Read the model definition and answer for the solid it produces. Units are mm, in the model's axes. Coordinates: 2 decimals unless noted, no trailing zeros. Write each loop counter-clockwise with the first axis right and the second up, starting at its lowest first coordinate (ties: lowest second). Pieces come first, ordered by that corner, then holes. Notation, with made-up numbers: M 54.25,50 L 78.25,50 A30 ccw 78.25,76 Z; hole C -7,-13 d8. An arc over 180 degrees is marked long. Write item = value, one per line.
Autodesk Inventor part; units mm, degrees
ref_plane "YZ Plane" through (0, 0, 0) normal (1, 0, 0) x (0, 1, 0)
ref_plane "XZ Plane" through (0, 0, 0) normal (0, 1, 0) x (-1, 0, 0)
ref_plane "XY Plane" through (0, 0, 0) normal (0, 0, 1) x (1, 0, 0)
sketch "Sketch1" plane through (0, 0, 0) normal (0, 1, 0) x (-1, 0, 0)
  line L0 (0, 0) -> (245, 0)
  line L1 (245, 0) -> (245, -355.6)
  line L2 (245, -355.6) -> (0, -355.6)
  line L3 (0, -355.6) -> (0, 0)
  line L4 (0, -355.6) -> (67.5, -355.6)
  line L5 (67.5, -355.6) -> (67.5, -280.6)
  line L6 (67.5, -280.6) -> (0, -280.6)
  line L7 (0, -280.6) -> (0, -355.6)
  line L8 (0, 0) -> (67.4878, 0)
  line L9 (67.4878, 0) -> (67.4878, -75.0062)
  line L10 (67.4878, -75.0062) -> (0, -75.0062)
  line L11 (0, -75.0062) -> (0, 0)
  dimension "d0" = 245
  dimension "d1" = 355.6
  dimension "d2" = 67.5
  dimension "d3" = 75
  dimension "d4" = 67.4878
  dimension "d5" = 75.0062
extrude "Extrusion1" add sketch "Sketch1" along normal blind 2.5 contours L0 L1 L2 L5 L6 L3 L10 L9
properties part number "Plexiglass Mounting Sheet" material "Acrylic, Clear"
Item 1: Find section C-C (z = -66). Determine the outline of the cut face in (x, y).
Worked answers:
outline = M -245,0 L -67.49,0 L -67.49,2.5 L -245,2.5 Z
Item 2: Find section B-B (x = -43.5). Determine the outline of the cut face in (y, z).
Worked answers:
outline = M 0,-280.6 L 2.5,-280.6 L 2.5,-75.01 L 0,-75.01 Z
Item 3: Find section A-A (y = 0.75). Determine the outline of the cut face in (x, z), and give its area (3 significant figures).
Worked answers:
outline = M -245,-355.6 L -67.5,-355.6 L -67.5,-280.6 L 0,-280.6 L 0,-75.01 L -67.49,-75.01 L -67.49,0 L -245,0 Z
area = 77,000 mm²
Item 4: Consider line 1 along Z through (x, y) = (-34, 0.8); line 2 along X through (y, z) = (0.5, -293.5). Determine where each line is inside the solid, lowest interval first. Write a range as from..to.
Worked answers:
line_1 = -280.6..-75.01
line_2 = -245..-67.5
